from build123d import *

# Parameters (mm, degrees)
F1_DEPTH = 40
F3_DEPTH = 26
F6_DEPTH = 376


with BuildPart() as f1:
    # F0 (on Top) → F1 (new body)
    with BuildSketch(Plane.XY):
        with BuildLine():
            Line((165, -135), (165, 25))
            Line((165, 25), (83.5, 25))
            ThreePointArc((83.5, 25), (83.4991991535, 24.6342942061), (83.4967966293, 24.2685954271))
            ThreePointArc((83.4967966293, 24.2685954271), (84.6154885355, 19.5843531992), (87.7939862549, 15.9662391769))
            ThreePointArc((87.7939862549, 15.9662391769), (92.2606519972, 4.5495209581), (83.3881264287, -3.9104345842))
            ThreePointArc((83.3881264287, -3.9104345842), (78.9784767448, -5.8465612578), (75.9852018745, -9.6193456912))
            ThreePointArc((75.9852018745, -9.6193456912), (72.1319392895, -17.0622554594), (67.5519565242, -24.0813933151))
            ThreePointArc((67.5519565242, -24.0813933151), (65.7426065331, -28.544559169), (66.2292845484, -33.3358785427))
            ThreePointArc((66.2292845484, -33.3358785427), (61.7955930136, -46.3209199003), (48.1502490008, -44.880952381))
            ThreePointArc((48.1502490008, -44.880952381), (44.922849365, -42.7482305425), (41.1274887886, -42))
            Line((41.1274887886, -42), (-41.1274887886, -42))
            ThreePointArc((-41.1274887886, -42), (-44.922849365, -42.7482305425), (-48.1502490008, -44.880952381))
            ThreePointArc((-48.1502490008, -44.880952381), (-61.7955930136, -46.3209199003), (-66.2292845484, -33.3358785427))
            ThreePointArc((-66.2292845484, -33.3358785427), (-65.7426065331, -28.544559169), (-67.5519565242, -24.0813933151))
            ThreePointArc((-67.5519565242, -24.0813933151), (-72.1319392895, -17.0622554594), (-75.9852018745, -9.6193456912))
            ThreePointArc((-75.9852018745, -9.6193456912), (-78.9784767448, -5.8465612578), (-83.3881264287, -3.9104345842))
            ThreePointArc((-83.3881264287, -3.9104345842), (-92.2606519972, 4.5495209581), (-87.7939862549, 15.9662391769))
            ThreePointArc((-87.7939862549, 15.9662391769), (-84.6154885355, 19.5843531992), (-83.4967966293, 24.2685954271))
            ThreePointArc((-83.4967966293, 24.2685954271), (-83.4991991535, 24.6342942061), (-83.5, 25))
            Line((-83.5, 25), (-165, 25))
            Line((-165, 25), (-165, -135))
            Line((-165, -135), (165, -135))
        make_face()
        with BuildLine():
            Line((165, 25), (165, 135))
            Line((165, 135), (-165, 135))
            Line((-165, 135), (-165, 25))
            Line((-165, 25), (-83.5, 25))
            ThreePointArc((-83.5, 25), (-83.1151125621, 33.0079999869), (-81.9639984721, 40.9421753368))
            ThreePointArc((-81.9639984721, 40.9421753368), (-82.2099154551, 45.7518657289), (-84.6754899777, 49.8888379435))
            ThreePointArc((-84.6754899777, 49.8888379435), (-85.5373543192, 64.3910516772), (-71.2643792291, 67.1001466184))
            Line((-71.2643792291, 67.1001466184), (-45, 51.58))
            Line((-45, 51.58), (-45, 44.1040966114))
            Line((-45, 44.1040966114), (-45, 25))
            Line((-45, 25), (0, 25))
            Line((0, 25), (45, 25))
            Line((45, 25), (45, 44.1040966114))
            Line((45, 44.1040966114), (45, 51.58))
            Line((45, 51.58), (71.2643792291, 67.1001466184))
            ThreePointArc((71.2643792291, 67.1001466184), (85.5373543192, 64.3910516772), (84.6754899777, 49.8888379435))
            ThreePointArc((84.6754899777, 49.8888379435), (82.2099154551, 45.7518657289), (81.9639984721, 40.9421753368))
            ThreePointArc((81.9639984721, 40.9421753368), (83.1151125621, 33.0079999869), (83.5, 25))
            Line((83.5, 25), (165, 25))
        make_face()
        with BuildLine():
            Line((0, 25), (-45, 25))
            ThreePointArc((-45, 25), (-44.7326165754, 20.1017335398), (-43.9336438082, 15.2616766467))
            Line((-43.9336438082, 15.2616766467), (0, 25))
        make_face()
        with BuildLine():
            Line((-30.1124291681, -8.4401197605), (0, 25))
            Line((0, 25), (-43.9336438082, 15.2616766467))
            ThreePointArc((-43.9336438082, 15.2616766467), (-38.8735002159, 2.3317186147), (-30.1124291681, -8.4401197605))
        make_face()
        with BuildLine():
            Line((30.1124291681, -8.4401197605), (0, 25))
            Line((0, 25), (-30.1124291681, -8.4401197605))
            ThreePointArc((-30.1124291681, -8.4401197605), (0, -20), (30.1124291681, -8.4401197605))
        make_face()
        with BuildLine():
            ThreePointArc((30.1124291681, -8.4401197605), (38.8735002159, 2.3317186147), (43.9336438082, 15.2616766467))
            Line((43.9336438082, 15.2616766467), (0, 25))
            Line((0, 25), (30.1124291681, -8.4401197605))
        make_face()
        with BuildLine():
            ThreePointArc((43.9336438082, 15.2616766467), (44.7326165754, 20.1017335398), (45, 25))
            Line((45, 25), (0, 25))
            Line((0, 25), (43.9336438082, 15.2616766467))
        make_face()
    extrude(amount=F1_DEPTH)

    # F2 (on face) → F3 (cut)
    with BuildSketch(Plane(origin=(0, 0, 0), x_dir=(1, 0, 0), z_dir=(0, 0, -1))):
        with BuildLine():
            Line((41.1274887886, 44), (-41.1274887886, 44))
            ThreePointArc((-41.1274887886, 44), (-44.1637772497, 44.598584434), (-46.7456969583, 46.3047619048))
            ThreePointArc((-46.7456969583, 46.3047619048), (-62.8720126099, 48.0065417003), (-68.1118298783, 32.6605837322))
            ThreePointArc((-68.1118298783, 32.6605837322), (-67.722487466, 28.8275282333), (-69.1699674589, 25.2569955502))
            ThreePointArc((-69.1699674589, 25.2569955502), (-73.8596504102, 18.0697346321), (-77.8052067098, 10.4485515761))
            ThreePointArc((-77.8052067098, 10.4485515761), (-80.1998266061, 7.4303240293), (-83.7275463532, 5.8814226904))
            ThreePointArc((-83.7275463532, 5.8814226904), (-94.2132583887, -4.1167065868), (-88.9344716024, -17.6091917545))
            ThreePointArc((-88.9344716024, -17.6091917545), (-86.3916734268, -20.5036829723), (-85.4967199018, -24.2510767547))
            ThreePointArc((-85.4967199018, -24.2510767547), (-85.1409902363, -32.8269905829), (-83.9272080163, -41.3240238478))
            ThreePointArc((-83.9272080163, -41.3240238478), (-84.1239416027, -45.1717761615), (-86.0964012208, -48.4813539332))
            ThreePointArc((-86.0964012208, -48.4813539332), (-87.1149681698, -65.6203338003), (-70.2469066998, -68.8219914581))
            Line((-70.2469066998, -68.8219914581), (-43, -52.7212497201))
            Line((-43, -52.7212497201), (-43, -25))
            ThreePointArc((-43, -25), (0, 18), (43, -25))
            Line((43, -25), (43, -52.7212497201))
            Line((43, -52.7212497201), (70.2469066998, -68.8219914581))
            ThreePointArc((70.2469066998, -68.8219914581), (87.1149681698, -65.6203338003), (86.0964012208, -48.4813539332))
            ThreePointArc((86.0964012208, -48.4813539332), (84.1239416027, -45.1717761615), (83.9272080163, -41.3240238478))
            ThreePointArc((83.9272080163, -41.3240238478), (85.1409902363, -32.8269905829), (85.4967199018, -24.2510767547))
            ThreePointArc((85.4967199018, -24.2510767547), (86.3916734268, -20.5036829723), (88.9344716024, -17.6091917545))
            ThreePointArc((88.9344716024, -17.6091917545), (94.2132583887, -4.1167065868), (83.7275463532, 5.8814226904))
            ThreePointArc((83.7275463532, 5.8814226904), (80.1998266061, 7.4303240293), (77.8052067098, 10.4485515761))
            ThreePointArc((77.8052067098, 10.4485515761), (73.8596504102, 18.0697346321), (69.1699674589, 25.2569955502))
            ThreePointArc((69.1699674589, 25.2569955502), (67.722487466, 28.8275282333), (68.1118298783, 32.6605837322))
            ThreePointArc((68.1118298783, 32.6605837322), (62.8720126099, 48.0065417003), (46.7456969583, 46.3047619048))
            ThreePointArc((46.7456969583, 46.3047619048), (44.1637772497, 44.598584434), (41.1274887886, 44))
        make_face()
        with BuildLine():
            Line((-45, -51.58), (-71.2643792291, -67.1001466184))
            ThreePointArc((-71.2643792291, -67.1001466184), (-85.5373543192, -64.3910516772), (-84.6754899777, -49.8888379435))
            ThreePointArc((-84.6754899777, -49.8888379435), (-82.2099154551, -45.7518657289), (-81.9639984721, -40.9421753368))
            ThreePointArc((-81.9639984721, -40.9421753368), (-83.1493881255, -32.6439030838), (-83.4967966293, -24.2685954271))
            ThreePointArc((-83.4967966293, -24.2685954271), (-84.6154885355, -19.5843531992), (-87.7939862549, -15.9662391769))
            ThreePointArc((-87.7939862549, -15.9662391769), (-92.2606519972, -4.5495209581), (-83.3881264287, 3.9104345842))
            ThreePointArc((-83.3881264287, 3.9104345842), (-78.9784767448, 5.8465612578), (-75.9852018745, 9.6193456912))
            ThreePointArc((-75.9852018745, 9.6193456912), (-72.1319392895, 17.0622554594), (-67.5519565242, 24.0813933151))
            ThreePointArc((-67.5519565242, 24.0813933151), (-65.7426065331, 28.544559169), (-66.2292845484, 33.3358785427))
            ThreePointArc((-66.2292845484, 33.3358785427), (-61.7955930136, 46.3209199003), (-48.1502490008, 44.880952381))
            ThreePointArc((-48.1502490008, 44.880952381), (-44.922849365, 42.7482305425), (-41.1274887886, 42))
            Line((-41.1274887886, 42), (41.1274887886, 42))
            ThreePointArc((41.1274887886, 42), (44.922849365, 42.7482305425), (48.1502490008, 44.880952381))
            ThreePointArc((48.1502490008, 44.880952381), (61.7955930136, 46.3209199003), (66.2292845484, 33.3358785427))
            ThreePointArc((66.2292845484, 33.3358785427), (65.7426065331, 28.544559169), (67.5519565242, 24.0813933151))
            ThreePointArc((67.5519565242, 24.0813933151), (72.1319392895, 17.0622554594), (75.9852018745, 9.6193456912))
            ThreePointArc((75.9852018745, 9.6193456912), (78.9784767448, 5.8465612578), (83.3881264287, 3.9104345842))
            ThreePointArc((83.3881264287, 3.9104345842), (92.2606519972, -4.5495209581), (87.7939862549, -15.9662391769))
            ThreePointArc((87.7939862549, -15.9662391769), (84.6154885355, -19.5843531992), (83.4967966293, -24.2685954271))
            ThreePointArc((83.4967966293, -24.2685954271), (83.1493881255, -32.6439030838), (81.9639984721, -40.9421753368))
            ThreePointArc((81.9639984721, -40.9421753368), (82.2099154551, -45.7518657289), (84.6754899777, -49.8888379435))
            ThreePointArc((84.6754899777, -49.8888379435), (85.5373543192, -64.3910516772), (71.2643792291, -67.1001466184))
            Line((71.2643792291, -67.1001466184), (45, -51.58))
            Line((45, -51.58), (45, -25))
            ThreePointArc((45, -25), (0, 20), (-45, -25))
            Line((-45, -25), (-45, -51.58))
        make_face(mode=Mode.SUBTRACT)
    extrude(amount=-F3_DEPTH, mode=Mode.SUBTRACT)

    # F5 (on face) → F6 (cut)
    with BuildSketch(Plane.YZ.offset(165)):
        Polygon((10.29, 40), (-48.05, 40), (10.29, 39), align=None)
        Polygon((68.63, 40), (10.29, 40), (10.29, 39), align=None)
    extrude(amount=-F6_DEPTH, mode=Mode.SUBTRACT)


solid = f1.part
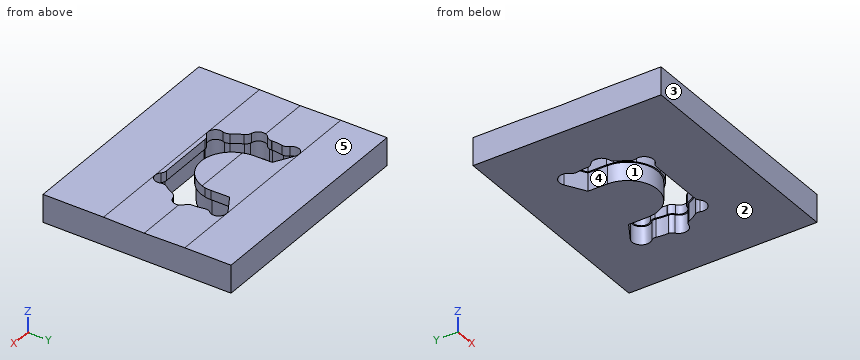
The listing builds one solid part. Answer for the finished solid, in the listing's coordinates (mm). Face numbers are marked on the shaded views. A direction names the side the tool comes from. Give positions to 0.01 mm unless a question says otherwise; leave off trailing zeros. Order: outer loops, then holes, each group sorted by start corner. A loop starts at its lowest first (then second) coordinate and runs counter-clockwise, first axis right, second up. Notation, with made-up numbers: (57, 30.25) - (95, 30.25) arc R20 ccw to (95, 65.25) - close; hole circle Ø9 at (25.5, 83). An arc over 180 degrees is marked (long way). One line per item, written item: value. Start each with the question number.
1) Find the intervals of material crossed by L1, parallel to X at y = 46, z = 33; L2, parallel to X at y = 63, z = 11; L3, parallel to Y at x = -87, z = 18, in increasing order.
2) A tool of negligible diameter and unlimited length cuts with its end or side. For the marked faces 4 and 5, from which of +Z, -Z, +X, -X, +Y, -Y can it reach the whole face along a straight path? Write none if from no direction.
3) The mould has two halves that part along Y. Classify the marked faces 1, 2 and 3: released by +Y, released by -Y, zero draft, split by the parting line, or undercut.
4) A cutting plane is placed at A-A on x = 0. Give the vertices of the cut face in (y, z).
5) A cutting plane is placed at C-C on x = -61.5. Give the vertices of the cut face in (y, z).
Answer sheet:
1. L1: x = -165 to -82.29, -45 to 45, 82.29 to 165
1. L2: x = -165 to -88.7, -60.39 to 60.39, 88.7 to 165
1. L3: y = -135 to -4.86, 19.51 to 49.49, 65.77 to 135
2. face 4: -Z
2. face 5: +Z, +X, -X, +Y, -Y
3. face 1: undercut
3. face 2: zero draft
3. face 3: released by -Y
4. outline: (-135, 0) - (-44, 0) - (-44, 26) - (-42, 26) - (-42, 39.9) - (-48.05, 40) - (-135, 40) - close; (-20, 26) - (-18, 26) - (-18, 0) - (135, 0) - (135, 40) - (68.63, 40) - (10.29, 39) - (-20, 39.52) - close
5. outline: (-135, 0) - (-48.77, 0) - (-48.77, 26) - (-46.5, 26) - (-46.5, 39.97) - (-48.05, 40) - (-135, 40) - close; (61.33, 26) - (63.65, 26) - (63.65, 0) - (135, 0) - (135, 40) - (68.63, 40) - (61.33, 39.87) - close
